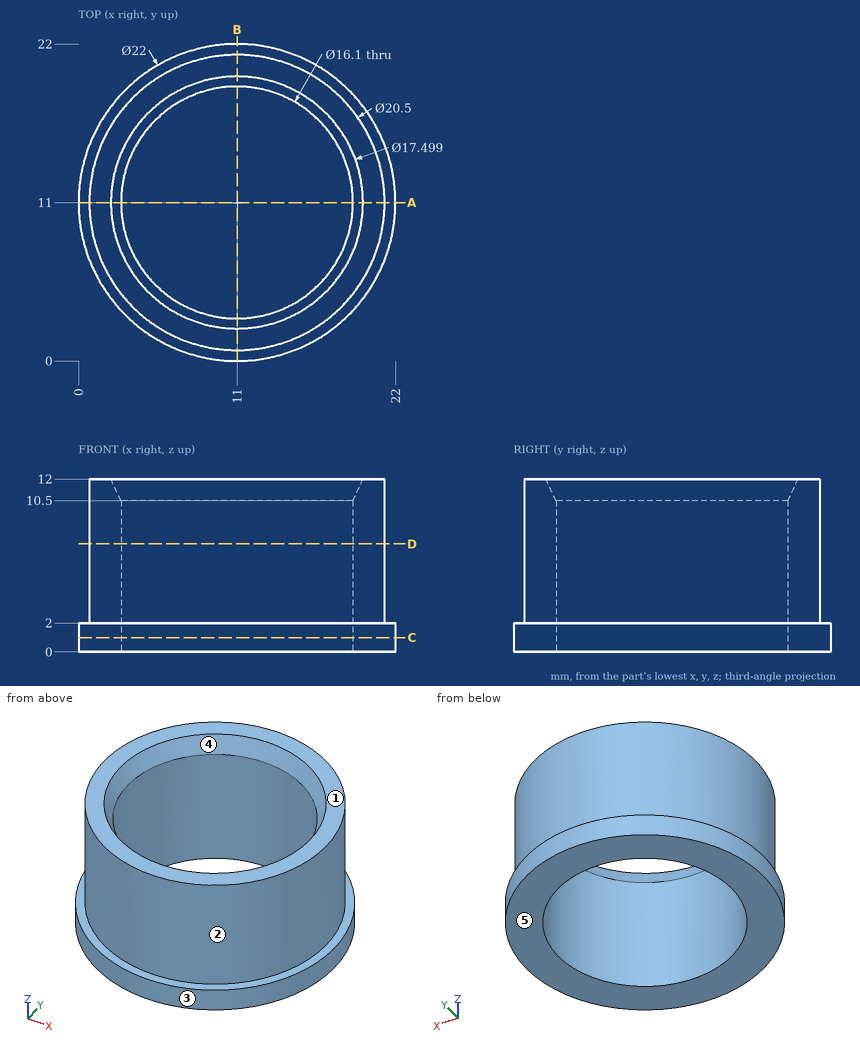
The drawing under review shows one solid part. Ordinate dimensions are in mm from its lowest x, y, z. A direction names the side the tool comes from. Round coordinates to 2 decimals unless told otherwise and drop trailing zeros. Order: outer loops, then holes, each group sorted by start corner. A loop starts at its lowest first (then second) coordinate and runs counter-clockwise, first axis right, second up. Notation, with made-up numbers: (48.25, -31.5) -> (67.25, -31.5) arc R13 cw to (67.25, -19.5) -> close; hole circle Ø8 at (35, 42). An arc over 180 degrees is marked (long way). Use a Markdown table: item, result.
Item 1: Draft analysis for pull direction X (two halves, no side actions). For the marked faces 3, 4 and 5, state which applies: +X half, -X half, draft (parallel to the pull), parting line (faces both ways), or undercut.
Resolved:
| item | result |
|---|---|
| face 3 | parting line |
| face 4 | undercut |
| face 5 | draft |
Item 2: Take a section at C-C (z = 1). State the section outline as (x, y) points, plus the area to 3 significant figures.
Resolved:
| item | result |
|---|---|
| outline | circle Ø22 at (11, 11); hole circle Ø16.1 at (11, 11) |
| area | 177 mm² |
Item 3: For line 1 along Y through (x, z) = (11, 6.25); line 2 along Y through (x, z) = (13.75, 10.75); line 3 along X through (y, z) = (9, 11.5), list the stretches that pass through material, from the lowest coordinate up. Write a range as [from, to].
Resolved:
| item | result |
|---|---|
| line 1 | y = [0.75, 2.95], [19.05, 21.25] |
| line 2 | y = [1.13, 3.31], [18.69, 20.87] |
| line 3 | x = [0.95, 2.72], [19.28, 21.05] |
Item 4: Take a section at D-D (z = 7.5). State the section outline as (x, y) points, plus the area to 3 significant figures.
Resolved:
| item | result |
|---|---|
| outline | circle Ø20.5 at (11, 11); hole circle Ø16.1 at (11, 11) |
| area | 126 mm² |
Item 5: Take a section at A-A (y = 11). State the section outline as (x, z) points.
Resolved:
| item | result |
|---|---|
| outline | (0, 0) -> (2.95, 0) -> (2.95, 10.5) -> (2.25, 12) -> (0.75, 12) -> (0.75, 2) -> (0, 2) -> close; (19.05, 0) -> (22, 0) -> (22, 2) -> (21.25, 2) -> (21.25, 12) -> (19.75, 12) -> (19.05, 10.5) -> close |
Item 6: Machinability: for the marked faces 1 and 2, which of the approach directions +Z, -Z, +X, -X, +Y, -Y give a long, thin tool a straight path to every point of the face, cutting with its end or side? Answer none if there is none.
Resolved:
| item | result |
|---|---|
| face 1 | +Z, +X, -X, +Y, -Y |
| face 2 | +Z |
Item 7: For pin 1 (4 mm diameter, centred on y = 13.5, z = 7, fed in from +X); pin 2 (2 mm diameter, centred on x = 11, z = 3.5, fed in from +Y); pin 3 (1 mm diameter, centred on y = 16, z = 2, fed in from +X), all flat-tipped, find the tip position at first contact; note any pin that passes through.
Resolved:
| item | result |
|---|---|
| pin 1 | stops at x = 21.24 |
| pin 2 | stops at y = 21.25 |
| pin 3 | stops at x = 21.04 |
